```python
from build123d import *

# Parameters (mm, degrees)
SKETCH1_R          = 9
EXTRUDE1_DEPTH     = 2
SKETCH4_R          = 7
EXTRUDE2_DEPTH     = 19
SKETCH2_R          = 5.5
CUT_EXTRUDE1_DEPTH = 10
SKETCH3_R          = 7.8
SKETCH3_R_2        = 7
CUT_EXTRUDE2_DEPTH = 1
SKETCH5_R          = 5
EXTRUDE3_DEPTH     = 8.5
SKETCH6_R          = 0.35
CUT_EXTRUDE3_DEPTH = 7
CHAMFER2_SIZE      = 0.15
CHAMFER1_SIZE      = 0.2
SKETCH7_R          = 5
CUT_EXTRUDE4_DEPTH = 1
CHAMFER3_SIZE      = 0.5
EXTRUDE4_DEPTH     = 3


with BuildPart() as part:
    # Sketch1 → Extrude1 (new body)
    with BuildSketch(Plane.XY):
        Circle(SKETCH1_R)
    extrude(amount=EXTRUDE1_DEPTH)

    # Sketch4 → Extrude2 (add)
    with BuildSketch(Plane(origin=(0, 0, 0), x_dir=(-1, 0, 0), z_dir=(0, 0, -1))):
        Circle(SKETCH4_R)
    extrude(amount=EXTRUDE2_DEPTH)

    # Sketch2 → Cut-Extrude1 (cut)
    with BuildSketch(Plane.XY.offset(2)):
        Circle(SKETCH2_R)
    extrude(amount=-CUT_EXTRUDE1_DEPTH, mode=Mode.SUBTRACT)

    # Sketch3 → Cut-Extrude2 (cut)
    with BuildSketch(Plane(origin=(0, 0, 0), x_dir=(-1, 0, 0), z_dir=(0, 0, -1))):
        Circle(SKETCH3_R)
        Circle(SKETCH3_R_2, mode=Mode.SUBTRACT)
    extrude(amount=-CUT_EXTRUDE2_DEPTH, mode=Mode.SUBTRACT)

    # Sketch5 → Extrude3 (add)
    with BuildSketch(Plane.XY.offset(-8)):
        Circle(SKETCH5_R)
    extrude(amount=EXTRUDE3_DEPTH)

    # Sketch6 → Cut-Extrude3 (cut)
    with BuildSketch(Plane.XY.offset(0.5)):
        with Locations((0, 3)):
            Circle(SKETCH6_R)
        with Locations((0, -3)):
            Circle(SKETCH6_R)
        with Locations((2.598076211, 1.5)):
            Circle(SKETCH6_R)
        with Locations((2.598076211, -1.5)):
            Circle(SKETCH6_R)
        with Locations((-2.598076211, 1.5)):
            Circle(SKETCH6_R)
        with Locations((-2.598076211, -1.5)):
            Circle(SKETCH6_R)
    extrude(amount=-CUT_EXTRUDE3_DEPTH, mode=Mode.SUBTRACT)

    # Chamfer2
    chamfer2_edges = [part.edges().sort_by_distance(p)[0] for p in [
        (-5, 0, 0.5),
        (-0.35, 3, 0.5),
        (-0.35, -3, 0.5),
        (2.248076211, 1.5, 0.5),
        (2.248076211, -1.5, 0.5),
        (-2.948076211, 1.5, 0.5),
        (-2.948076211, -1.5, 0.5),
    ]]
    chamfer(chamfer2_edges, length=CHAMFER2_SIZE)

    # Chamfer1
    chamfer1_edges = [part.edges().sort_by_distance(p)[0] for p in [
        (-5.5, 0, 2),
        (-9, 0, 2),
    ]]
    chamfer(chamfer1_edges, length=CHAMFER1_SIZE)

    # Sketch7 → Cut-Extrude4 (cut)
    with BuildSketch(Plane(origin=(0, 0, -19), x_dir=(-1, 0, 0), z_dir=(0, 0, -1))):
        Circle(SKETCH7_R)
    extrude(amount=-CUT_EXTRUDE4_DEPTH, mode=Mode.SUBTRACT)

    # Chamfer3
    chamfer3_edges = [part.edges().sort_by_distance(p)[0] for p in [
        (7, 0, -19),
    ]]
    chamfer(chamfer3_edges, length=CHAMFER3_SIZE)

    # Sketch8 → Extrude4 (add)
    with BuildSketch(Plane(origin=(0, 0, -18), x_dir=(-1, 0, 0), z_dir=(0, 0, -1))):
        Polygon((-4.907477288, 8.5), (4.907477288, 8.5), (9.814954576, 0), (4.907477288, -8.5), (-4.907477288, -8.5), (-9.814954576, 0), align=None)
    extrude(amount=-EXTRUDE4_DEPTH)


solid = part.part
```
The model under review builds one solid part; all positions refer to its coordinate system, in mm. A direction names the side the tool comes from. Round coordinates to 2 decimals unless told otherwise and drop trailing zeros. Order: outer loops, then holes, each group sorted by start corner. A loop starts at its lowest first (then second) coordinate and runs counter-clockwise, first axis right, second up. Notation, with made-up numbers: (55.25, 58) -> (82.25, 58) arc R11 ccw to (82.25, 71) -> close; hole circle Ø6 at (74, 36.5). An arc over 180 degrees is marked (long way). One line per item, written item: value. Start each with the question number.
Q1. Machinability: for faces 4 (the face through (5.04, 5.08, -15)), 5 (the face through (0, 0, -18)), 6 (the face through (-7.327, 4.309, -16.521)), 7 (the face through (-1.08, -4.88, -3.88)), which of the approach directions +Z, -Z, +X, -X, +Y, -Y give a long, thin tool a straight path to every point of the face, cutting with its end or side? Answer none if there is none.
Q2. Take a section at A-A (z = -2.75). Count the separate pieces of the cut face and the enclosed holes in it, and give its area (3 significant figures).
Q3. Take a section at B-B (z = -15.75). Write out the cut boundary in (x, y).
Q4. Mouldability with a two-part tool opening along Y and no side actions: class faces 1 (the face through (-7.396, -4.191, -16.521)), 2 (the face through (-1.19, -5.37, -3.03)), 3 (the face through (0, 8.5, -17)) as released by +Y, released by -Y, zero draft, split by the parting line, or undercut.
Q5. Wall thickness on line 1 (Y direction, x = 0, z = -2.25); line 2 (Y direction, x = 0, z = 0.8); line 3 (X direction, y = -1.25, z = -6.75): over which ranges is each line inside the solid? List them lowest first.
Q6. Clearance check with flat-ended pins moving along their axes: pin 1 Ø1.5 at (x, z) = (4, -10.5) entering from -Y; pin 2 Ø1.5 at (x, z) = (5.5, -16) entering from -Y; pin 3 Ø6 at (x, z) = (-0.5, -12.5) entering from +Y. State where each tip first meets the part, or that it passes through.
Reported:
1. face 4: none
1. face 5: -Z
1. face 6: -Z, -X, +Y
1. face 7: +Z
2. separate pieces: 2
2. enclosed holes: 7
2. area: 135 mm2
3. outline: (-9.81, 0) -> (-4.91, -8.5) -> (4.91, -8.5) -> (9.81, 0) -> (4.91, 8.5) -> (-4.91, 8.5) -> close
4. face 1: released by -Y
4. face 2: undercut
4. face 3: released by +Y
5. line 1: y = -7 to -5.5, -5 to -3.35, -2.65 to 2.65, 3.35 to 5, 5.5 to 7
5. line 2: y = -9 to -7.8, -7 to -5.5, 5.5 to 7, 7.8 to 9
5. line 3: x = -6.89 to -5.36, -4.84 to 4.84, 5.36 to 6.89
6. pin 1: stops at y = -6.2
6. pin 2: stops at y = -8.5
6. pin 3: stops at y = 8.5
